Here's the drawing with two shaded views (mm, measured from the low corner). I have some questions. A direction names the side the tool comes from. Round coordinates to 2 decimals unless told otherwise and drop trailing zeros. Loops run counter-clockwise (first coordinate to the right, second up) from the corner with the lowest first, then second, coordinate; pieces in that order, holes last.
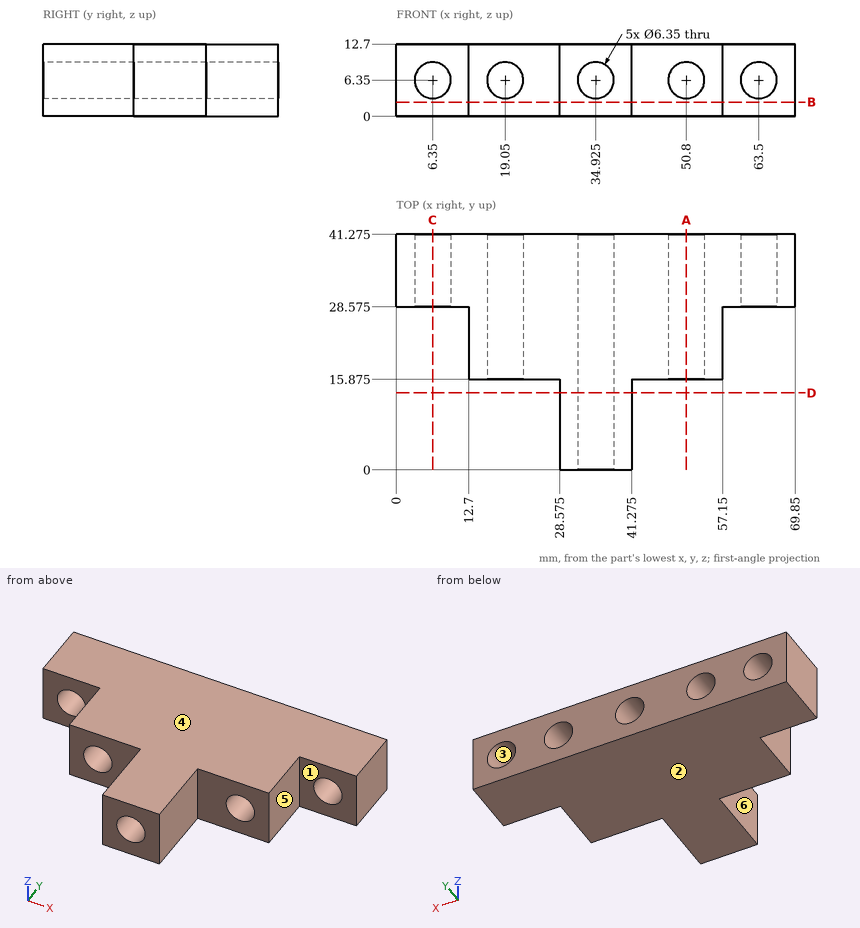
(1) If we section it at D-D, the plane y = 13.5: List the corners of the cut face in (x, z) for me (3 decimals).
Worked answers:
outline: (28.575, 0) - (41.275, 0) - (41.275, 12.7) - (28.575, 12.7) - close; hole circle Ø6.35 at (34.925, 6.35)
(2) For the marked faces 4, 5 and 6, which set-ups out of +Z, -Z, +X, -X, +Y, -Y let a thin tool reach every point of the face, with its end or its side?
Worked answers:
face 4: +Z, +X, -X, +Y, -Y
face 5: +Z, -Z, +X, -Y
face 6: +Z, -Z, -X, -Y
(3) If we section it at C-C, the plane x = 6.35: List the corners of the cut face in (y, z) for me (3 decimals).
Worked answers:
outline: (28.575, 0) - (41.275, 0) - (41.275, 3.175) - (28.575, 3.175) - close; (28.575, 9.525) - (41.275, 9.525) - (41.275, 12.7) - (28.575, 12.7) - close
(4) If we section it at B-B, the plane z = 2.5: List the corners of the cut face in (x, y) for me (3 decimals).
Worked answers:
outline: (0, 28.575) - (12.7, 28.575) - (12.7, 15.875) - (28.575, 15.875) - (28.575, 0) - (41.275, 0) - (41.275, 15.875) - (57.15, 15.875) - (57.15, 28.575) - (69.85, 28.575) - (69.85, 41.275) - (0, 41.275) - close
(5) If I drill on line 1 (X direction, y = 37.75, z = 6.35) (3 decimals); line 2 (X direction, y = 21, z = 6.35) (3 decimals); line 3 (X direction, y = 20.5, z = 4.75), over which ranges is the centre line in solid material (lowest first)?
Worked answers:
line 1: x = 0 to 3.175, 9.525 to 15.875, 22.225 to 31.75, 38.1 to 47.625, 53.975 to 60.325, 66.675 to 69.85
line 2: x = 12.7 to 15.875, 22.225 to 31.75, 38.1 to 47.625, 53.975 to 57.15
line 3: x = 12.7 to 16.31, 21.79 to 32.18, 37.67 to 48.06, 53.54 to 57.15
(6) If we section it at A-A, the plane x = 50.8: List the corners of the cut face in (y, z) for me (3 decimals).
Worked answers:
outline: (15.875, 0) - (41.275, 0) - (41.275, 3.175) - (15.875, 3.175) - close; (15.875, 9.525) - (41.275, 9.525) - (41.275, 12.7) - (15.875, 12.7) - close
(7) If we mould it in two halves opening along Z, with no side actions, what happens to the marked faces 1, 2 and 3? For each: released by +Z, released by -Z, zero draft, split by the parting line, or undercut.
Worked answers:
face 1: zero draft
face 2: released by -Z
face 3: undercut
(8) Will these pins go through, and if not, where does the flat tip stop? P1, Ø6, axis at x = 19.5, z = 4, coming from the -Y side (3 decimals); P2, Ø5.5, axis at x = 19.05, z = 6.35, coming from the -Y side; P3, Ø6.5, axis at y = 6.5, z = 4.5, coming from the -X side (3 decimals).
Worked answers:
P1: stops at y = 15.875
P2: passes through
P3: stops at x = 28.575
